For this review, take the finished solid that the model builds, in its own axes (mm). Round coordinates to 2 decimals unless told otherwise and drop trailing zeros. Loops run counter-clockwise (first coordinate to the right, second up) from the corner with the lowest first, then second, coordinate; pieces in that order, holes last.
1) Take a section at A-A (y = 25.75). State the section outline as (x, z) points.
2) Insertion check: pin 1 (3 mm diameter, centred on x = 1.5, y = 26, fed in from -Z); pin 2 (2 mm diameter, centred on x = -7.5, z = 3.5, fed in from +Y); pin 3 (1.5 mm diameter, centred on x = -4.5, y = 28, fed in from -Z). Each pin has a flat end and moves straight along its axis. Give the tip position at first contact, or say it passes through.
3) Wall thickness on L1, parallel to Z at x = -4.75, y = 26.5; L2, parallel to Z at x = -7.25, y = 26.3; L3, parallel to Y at x = -3.75, z = -7.5: over which ranges is each line inside the solid? List them lowest first.
4) Take a section at B-B (x = 3). State the section outline as (y, z) points, then the cut area to 3 significant figures.
5) Take a section at C-C (z = 14). State the section outline as (x, y) points.
```python
from build123d import *

# Parameters (mm, degrees)
BOX002_W        = 10
BOX002_H        = 10
BOX002_DEPTH    = 40
BOX001_W        = 10
BOX001_H        = 10
BOX001_DEPTH    = 40
BOX_W           = 60
BOX_H           = 40
BOX_DEPTH       = 60
SPHERE001_ANGLE = 180
SPHERE_ANGLE    = 180


with BuildPart() as cube002:
    # Box002 → Box002 (new body)
    with BuildSketch(Plane(origin=(-20, 20, -20), x_dir=(1, 0, 0), z_dir=(0, 0, 1))):
        with Locations((5, 5)):
            Rectangle(BOX002_W, BOX002_H)
    extrude(amount=BOX002_DEPTH)


with BuildPart() as cube001:
    # Box001 → Box001 (new body)
    with BuildSketch(Plane(origin=(10, 20, -20), x_dir=(1, 0, 0), z_dir=(0, 0, 1))):
        with Locations((5, 5)):
            Rectangle(BOX001_W, BOX001_H)
    extrude(amount=BOX001_DEPTH)


with BuildPart() as cube:
    # Box → Box (new body)
    with BuildSketch(Plane(origin=(-30, -15, -30), x_dir=(1, 0, 0), z_dir=(0, 0, 1))):
        with Locations((30, 20)):
            Rectangle(BOX_W, BOX_H)
    extrude(amount=BOX_DEPTH)


with BuildPart() as inner:
    # Sphere001 → Sphere001 (revolve)
    with BuildSketch(Plane.XZ):
        with BuildLine():
            ThreePointArc((0, -29.7), (29.7, 0), (0, 29.7))
            Line((0, 29.7), (0, -29.7))
        make_face()
    revolve(axis=Axis((0, 0, 0), (0, 0, 1)), revolution_arc=SPHERE001_ANGLE)


with BuildPart() as cutmirror:
    # Sphere → Sphere (revolve)
    with BuildSketch(Plane.XZ):
        with BuildLine():
            ThreePointArc((0, -30), (30, 0), (0, 30))
            Line((0, 30), (0, -30))
        make_face()
    revolve(axis=Axis((0, 0, 0), (0, 0, 1)), revolution_arc=SPHERE_ANGLE)

    # Cut: cut Inner
    add(inner.part, mode=Mode.SUBTRACT)

    # Cut001: cut Cube
    add(cube.part, mode=Mode.SUBTRACT)

    # Cut002: cut Cube001
    add(cube001.part, mode=Mode.SUBTRACT)

    # Cut003: cut Cube002
    add(cube002.part, mode=Mode.SUBTRACT)


solid = cutmirror.part
```
Response:
1. outline: (-10, -11.7) arc R15.39 ccw to (10, -11.7) - (10, -10.91) arc R14.8 cw to (-10, -10.91) - close; (-10, 10.91) arc R14.8 cw to (10, 10.91) - (10, 11.7) arc R15.39 ccw to (-10, 11.7) - close
2. pin 1: stops at z = -16.58
2. pin 2: stops at y = 29.1
2. pin 3: stops at z = -11.74
3. L1: z = -13.24 to -12.54, 12.54 to 13.24
3. L2: z = -12.48 to -11.74, 11.74 to 12.48
3. L3: y = 28.49 to 28.8
4. outline: (25, -16.31) arc R29.85 ccw to (25, 16.31) - (25, 15.75) arc R29.55 cw to (25, -15.75) - close
4. area: 10.2 mm2
5. outline: (-8.89, 25) - (-7.82, 25) arc R26.19 cw to (7.82, 25) - (8.89, 25) arc R26.53 ccw to start
